```python
from build123d import *

# Parameters (mm, degrees)
SKETCH1_R                                           = 79
BOSS_EXTRUDE1_DEPTH                                 = 29
CBORE_FOR_00_BINDING_HEAD_MACHINE_SCREW_D           = 96.000000024
CBORE_FOR_00_BINDING_HEAD_MACHINE_SCREW_CBORE_D     = 112.000000028
CBORE_FOR_00_BINDING_HEAD_MACHINE_SCREW_CBORE_DEPTH = 11.999999876
TAP_DRILL_FOR_M12X1_5_TAP2_D                        = 10.5


with BuildPart() as part:
    # Sketch1 → Boss-Extrude1 (new body)
    with BuildSketch(Plane(origin=(0, 0, 0), x_dir=(1, 0, 0), z_dir=(0, 1, 0))):
        Circle(SKETCH1_R)
    extrude(amount=BOSS_EXTRUDE1_DEPTH)

    # CBORE for #00 Binding Head Machine Screw1 (through all)
    with Locations(Plane(origin=(0, 29, 0), x_dir=(1, 0, 0), z_dir=(0, 1, 0))):
        with Locations((0, 0)):
            CounterBoreHole(CBORE_FOR_00_BINDING_HEAD_MACHINE_SCREW_D / 2, CBORE_FOR_00_BINDING_HEAD_MACHINE_SCREW_CBORE_D / 2, CBORE_FOR_00_BINDING_HEAD_MACHINE_SCREW_CBORE_DEPTH)

    # Tap Drill for M12x1.5 Tap2 (through all)
    with Locations(Plane(origin=(0, 29, 0), x_dir=(1, 0, 0), z_dir=(0, 1, 0))):
        with Locations((54.411006739, -33.696325403), (-1.976370444, -63.969476783), (-56.387377183, -30.27315138), (-54.411006739, 33.696325403), (1.976370444, 63.969476783), (56.387377183, 30.27315138), (0, 0)):
            Hole(TAP_DRILL_FOR_M12X1_5_TAP2_D / 2)


solid = part.part
```
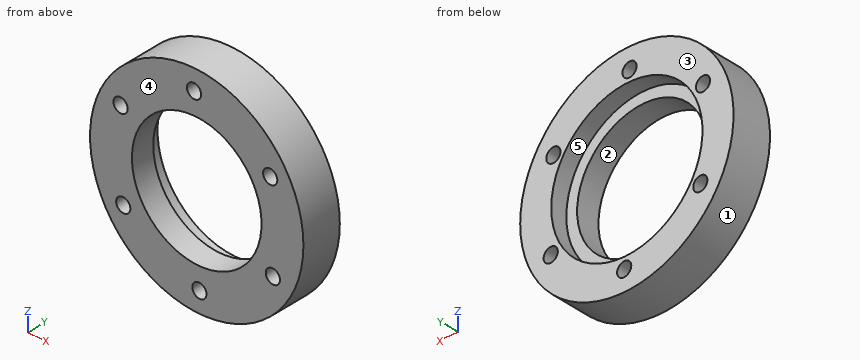
Input: part model. Units: mm. Frame: model coordinates. Face numbers are marked on the shaded views. A direction names the side the tool comes from. Round coordinates to 2 decimals unless told otherwise and drop trailing zeros. Loops run counter-clockwise (first coordinate to the right, second up) from the corner with the lowest first, then second, coordinate; pieces in that order, holes last.
1) Pin query (flat end, axial travel): pin 1 (8.5 mm diameter, centred on x = -1.98, z = 63.97, fed in from +Y); pin 2 (2 mm diameter, centred on y = 24.5, z = -41.5, fed in from -X); pin 3 (8 mm diameter, centred on x = -48.5, y = 4.5, fed in from -Z); pin 4 (10 mm diameter, centred on x = 33.5, y = 24, fed in from -Z). Return the tip coordinate at first contact, or that it passes through.
Ans:
pin 1: passes through
pin 2: stops at x = -67.83
pin 3: stops at z = -65.27
pin 4: stops at z = -73.68
2) Section query A-A on z = 0. Return the cut outline in (x, y), plus the area to 3 significant figures.
Ans:
outline: (-79, 0) - (-48, 0) - (-48, 17) - (-56, 17) - (-56, 29) - (-79, 29) - close; (48, 0) - (79, 0) - (79, 29) - (56, 29) - (56, 17) - (48, 17) - close
area: 1,610 mm2
3) Set-up query: the marked faces 4 and 5. Return all of +Z, -Z, +X, -X, +Y, -Y with unobstructed straight access to the full face (end or side cutting, diameter ignored); none if empty.
Ans:
face 4: +Z, -Z, +X, -X, -Y
face 5: +Y
4) Pull-direction query (X, two-part tool) for the marked faces 1, 2 and 3; classes: released by +X, released by -X, zero draft, split by the parting line, or undercut.
Ans:
face 1: split by the parting line
face 2: undercut
face 3: zero draft
5) Section query B-B on x = -19.5. Return the cut outline in (y, z).
Ans:
outline: (0, -76.56) - (29, -76.56) - (29, -52.5) - (17, -52.5) - (17, -43.86) - (0, -43.86) - close; (0, 43.86) - (17, 43.86) - (17, 52.5) - (29, 52.5) - (29, 76.56) - (0, 76.56) - close
6) Material intervals for line 1 (X direction, y = 14.75, z = -32); line 2 (X direction, y = 11.5, z = 32.5); line 3 (Z direction, x = 0, y = 13.25), sorted ascending.
Ans:
line 1: x = -72.23 to -59.38, -49.44 to -35.78, 35.78 to 51.43, 61.35 to 72.23
line 2: x = -72.01 to -61.14, -51.63 to -35.32, 35.32 to 49.3, 59.52 to 72.01
line 3: z = -79 to -68.83, -59.11 to -48, 48 to 59.11, 68.83 to 79
7) Section query D-D on x = 0. Return the cut outline in (y, z).
Ans:
outline: (0, -79) - (29, -79) - (29, -68.83) - (0, -68.83) - close; (0, -59.11) - (29, -59.11) - (29, -56) - (17, -56) - (17, -48) - (0, -48) - close; (0, 48) - (17, 48) - (17, 56) - (29, 56) - (29, 59.11) - (0, 59.11) - close; (0, 68.83) - (29, 68.83) - (29, 79) - (0, 79) - close
8) Section query C-C on y = 23.75. Return the cut outline in (x, z), plus the area to 3 significant figures.
Ans:
outline: circle Ø158 at (0, 0); hole circle Ø10.5 at (-56.39, 30.27); hole circle Ø10.5 at (-54.41, -33.7); hole circle Ø112 at (0, 0); hole circle Ø10.5 at (-1.98, 63.97); hole circle Ø10.5 at (1.98, -63.97); hole circle Ø10.5 at (54.41, 33.7); hole circle Ø10.5 at (56.39, -30.27)
area: 9,240 mm2
